Could you check a few things on this drawing? It's one solid part, dimensions in mm from its lowest x, y, z. A direction names the side the tool comes from. Give positions to 0.01 mm unless a question says otherwise; leave off trailing zeros. Loops run counter-clockwise (first coordinate to the right, second up) from the corner with the lowest first, then second, coordinate; pieces in that order, holes last. Notation, with made-up numbers: (51, 42) - (94, 42) arc R11 cw to (94, 60) - close; hole circle Ø5 at (43.5, 85.5). An arc over 180 degrees is marked (long way). Write item = value, one per line.
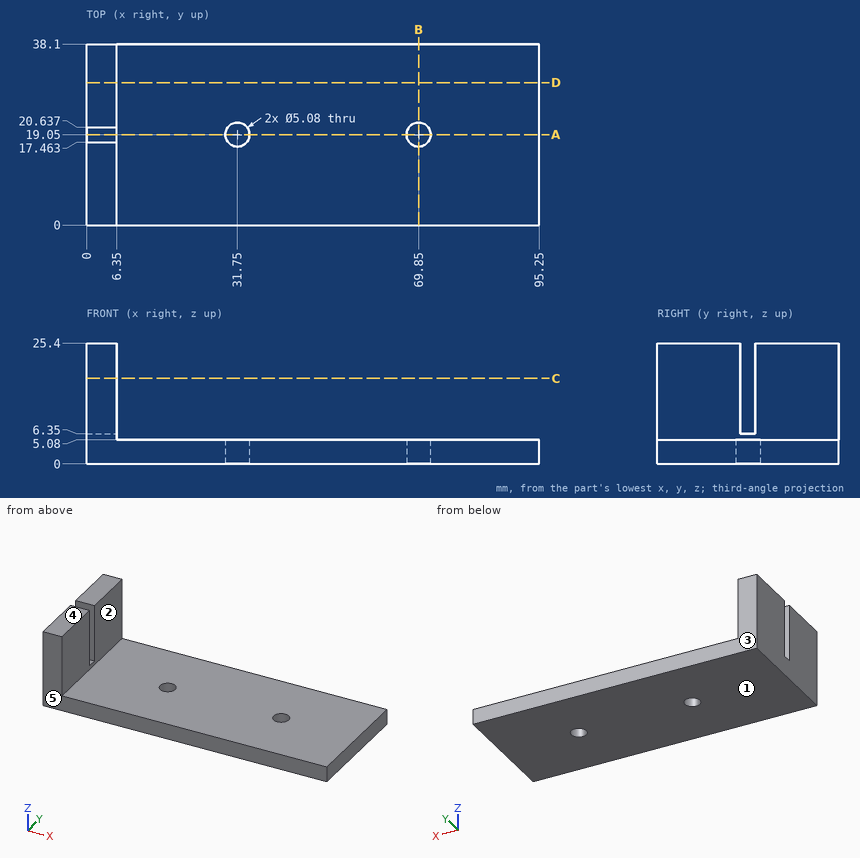
Q1. For pin 1 (8 mm diameter, centred on y = 25, z = 14, fed in from +X); pin 2 (6.5 mm diameter, centred on x = 31.75, y = 19.05, fed in from +Z), each with a flat end and sliding along its axis, tell me the tip position at first contact or that it passes through.
Output:
pin_1 = 6.35
pin_2 = 5.08
Q2. Which directions (+Z, -Z, +X, -X, +Y, -Y) give clear straight access to the entire face, cutting with the end or side of a thin tool? Please do the marked faces 1 and 2.
Output:
face_1 = -Z, +X, -X, +Y, -Y
face_2 = +Z, +X, +Y, -Y
Q3. Imagine slicing it at B-B, the plane x = 69.85. Write out the boundary of the cut face in (y, z).
Output:
outline = (0, 0) - (16.51, 0) - (16.51, 5.08) - (0, 5.08) - close; (21.59, 0) - (38.1, 0) - (38.1, 5.08) - (21.59, 5.08) - close
Q4. We'd pull the mould along Y, two halves only. Please class the marked faces 3, 4 and 5: released by +Y, released by -Y, zero draft, split by the parting line, or undercut.
Output:
face_3 = released by +Y
face_4 = zero draft
face_5 = released by -Y
Q5. Imagine slicing it at C-C, the plane z = 18. Write out the boundary of the cut face in (x, y), then the cut area to 3 significant figures.
Output:
outline = (0, 0) - (6.35, 0) - (6.35, 17.46) - (0, 17.46) - close; (0, 20.64) - (6.35, 20.64) - (6.35, 38.1) - (0, 38.1) - close
area = 222 mm2
Q6. Imagine slicing it at A-A, the plane y = 19.05. Write out the boundary of the cut face in (x, z).
Output:
outline = (0, 0) - (29.21, 0) - (29.21, 5.08) - (6.35, 5.08) - (6.35, 6.35) - (0, 6.35) - close; (34.29, 0) - (67.31, 0) - (67.31, 5.08) - (34.29, 5.08) - close; (72.39, 0) - (95.25, 0) - (95.25, 5.08) - (72.39, 5.08) - close
Q7. I need wall thicknesses on L1, parallel to X at y = 19.05, z = 2.6; L2, parallel to Y at x = 31.75, z = 4; L3, parallel to Z at x = 29.5, y = 8. Which ranges of each line are inside material? Lowest first, please.
Output:
L1 = 0 to 29.21, 34.29 to 67.31, 72.39 to 95.25
L2 = 0 to 16.51, 21.59 to 38.1
L3 = 0 to 5.08
Q8. Imagine slicing it at D-D, the plane y = 30. Write out the boundary of the cut face in (x, z).
Output:
outline = (0, 0) - (95.25, 0) - (95.25, 5.08) - (6.35, 5.08) - (6.35, 25.4) - (0, 25.4) - close
